Autodesk Inventor part; units mm, degrees
ref_plane "YZ Plane" through (0, 0, 0) normal (1, 0, 0) x (0, 1, 0)
ref_plane "XZ Plane" through (0, 0, 0) normal (0, 1, 0) x (-1, 0, 0)
ref_plane "XY Plane" through (0, 0, 0) normal (0, 0, 1) x (1, 0, 0)
ref_plane "Work Plane1" through (0, 0, 0) normal (0, 0, 1) x (1, 0, 0)
sketch "Sketch1" plane through (0, 0, 0) normal (0, 0, 1) x (1, 0, 0)
  circle A0 centre (103.8623, 15.35) radius 2.15 construction
  circle A1 centre (103.8623, -15.35) radius 2.15 construction
  line L0 (-103.8623, 20.35) -> (-103.8623, -20.35) construction
  line L1 (108.8623, -20.35) -> (-103.8623, -20.35) construction
  line L2 (108.8623, 20.35) -> (108.8623, -20.35) construction
  line L3 (-103.8623, 20.35) -> (108.8623, 20.35) construction
  circle A2 centre (59.3407, 0) radius 6.5 construction
  circle A3 centre (59.3407, 0) radius 7
  circle A4 centre (59.3407, 0) radius 24.5216 construction
  line L4 (34.8192, 0) -> (24.8192, 0) construction
  line L5 (24.8192, -20.35) -> (24.8192, 20.35)
  line L6 (24.8192, 20.35) -> (98.3623, 20.35)
  line L7 (98.8623, -20.35) -> (98.8623, 20.35) construction
  line L8 (98.3623, -20.35) -> (24.8192, -20.35)
  line L9 (95.8623, -23.35) -> (95.8623, 9.65)
  line L10 (95.3623, -20.35) -> (24.8192, -20.35)
  line L11 (98.8623, 9.65) -> (95.8623, 9.65)
  line L12 (98.8623, 20.35) -> (98.8623, -20.35)
  line L13 (98.3623, 10.15) -> (95.3623, 10.15)
  line L14 (95.3623, 10.15) -> (95.3623, -23.3504)
  line L15 (98.3623, 10.15) -> (98.3623, 20.35)
  point P0 (0, 0)
  point P1 (95.3623, -20.35)
  dimension "d0" = 0.5
  dimension "d1" = 10
  dimension "d15" = 0.5
  dimension "d16" = 0.5
  dimension "d17" = 0.5
extrude "Extrusion1" add sketch "Sketch1" along normal blind 5
sketch "Sketch2" plane through (24.8192, -20.35, 0) normal (-1, 0, 0) x (0, 0, 1)
  line L0 (80.8, 35.7) -> (75.8, 35.7) construction
  line L1 (80.8, 45.7) -> (80.8, 35.7) construction
  line L2 (51.1, 45.7) -> (80.8, 45.7) construction
  line L3 (51.1, -4.2229) -> (51.1, 45.7) construction
  line L4 (26.6, -4.2229) -> (51.1, -4.2229) construction
  line L5 (26.6, -16.2229) -> (26.6, -4.2229) construction
  line L6 (65.2, -16.2229) -> (26.6, -16.2229) construction
  line L7 (65.2, 40.7) -> (65.2, -16.2229) construction
  line L8 (75.8, 40.7) -> (65.2, 40.7) construction
  line L9 (75.8, 35.7) -> (75.8, 40.7) construction
  line L10 (38.6, -16.2229) -> (0, -16.2229)
  line L11 (0, -16.2229) -> (0, -4.2229)
  line L12 (5, -4.2229) -> (38.6, -4.2229)
  line L13 (38.6, -4.2229) -> (38.6, -16.2229)
  line L14 (38.6, -10.2229) -> (26.6, -10.2229) construction
  line L15 (0, 40.7) -> (0, 0) construction
  line L16 (0, 0) -> (5, 0) construction
  line L17 (5, 40.7) -> (5, 0) construction
  line L18 (0, 40.7) -> (5, 40.7) construction
  line L19 (5, 5) -> (0, 5)
  line L20 (0, -4.2229) -> (0, 5)
  line L21 (5, 5) -> (5, -4.2229)
  point P0 (0, 20.35)
  dimension "d11" = 5
extrude "Extrusion2" add sketch "Sketch2" against normal blind 5
equation "\"d15\" = d0"
equation "\"d16\" = d0"
equation "\"d17\" = d0"
equation "\"d9\" = d2"
equation "\"d11\" = d2"
equation "\"d12\" = d2"
properties part number "Button Bracket 2"
Here's how the part is built. I have some questions about the finished solid (model axes, mm). A direction names the side the tool comes from. Coordinates: 2 decimals unless noted, no trailing zeros. Order: outer loops, then holes, each group sorted by start corner. A loop starts at its lowest first (then second) coordinate and runs counter-clockwise, first axis right, second up. Notation, with made-up numbers: (41, 52.5) -> (51, 52.5) arc R9 ccw to (51, 62.5) -> close; hole circle Ø8 at (-10.75, 31). An arc over 180 degrees is marked (long way). Return JSON: item names as keys, results as strings.
1) If we section it at C-C on x = 57: List the corners of the cut face in (y, z) for me, plus the area to 3 significant figures.
Conclusion:
{"outline": "(-20.35, 0) -> (-6.6, 0) -> (-6.6, 5) -> (-20.35, 5) -> close; (6.6, 0) -> (20.35, 0) -> (20.35, 5) -> (6.6, 5) -> close", "area": "138 mm²"}
2) If I drill on probe 1 along X at (y, z) = (-29, 10); probe 2 along Y at (x, z) = (31, 3); probe 3 along Z at (x, y) = (74, -9.5), over which ranges is the centre line in solid material (lowest first)?
Conclusion:
{"probe 1": "x = 24.82 to 29.82", "probe 2": "y = -20.35 to 20.35", "probe 3": "z = 0 to 5"}
3) If we section it at D-D on z = 22: List the corners of the cut face in (x, y) for me, plus the area to 3 significant figures.
Conclusion:
{"outline": "(24.82, -36.57) -> (29.82, -36.57) -> (29.82, -24.57) -> (24.82, -24.57) -> close", "area": "60.0 mm²"}
4) I'm going to push flat-ended pins straight in: P1, Ø8, axis at y = -30.5, z = 24, coming from the +X side; P2, Ø1.5, axis at x = 63, y = -18.5, coming from the +Z side; P3, Ø1.5, axis at x = 97, z = 3.5, coming from the -Y side; P4, Ø5, axis at x = 33.5, z = 28, coming from the -Y side. Where does each tip first touch, or does it pass through?
Conclusion:
{"P1": "stops at x = 29.82", "P2": "stops at z = 5", "P3": "stops at y = 10.15", "P4": "passes through"}
5) If we section it at B-B on z = 4: List the corners of the cut face in (x, y) for me.
Conclusion:
{"outline": "(24.82, -36.57) -> (29.82, -36.57) -> (29.82, -20.35) -> (95.36, -20.35) -> (95.36, 10.15) -> (98.36, 10.15) -> (98.36, 20.35) -> (24.82, 20.35) -> close; hole circle Ø14 at (59.34, 0)"}
6) If we section it at A-A on y = 0: List the corners of the cut face in (x, z) for me, plus the area to 3 significant figures.
Conclusion:
{"outline": "(24.82, 0) -> (52.34, 0) -> (52.34, 5) -> (24.82, 5) -> close; (66.34, 0) -> (95.36, 0) -> (95.36, 5) -> (66.34, 5) -> close", "area": "283 mm²"}
7) Thinking about a two-plate mould opening in X: for faces 4 (the flat face through (24.819, -25, 15)), 5 (the flat face through (95.362, -5, 2)), 6 (the cylindrical face through (52.347, -0.308, 2.465)), 7 (the flat face through (27, -36.573, 20)), which applies, +X half, -X half, draft (parallel to the pull), parting line (faces both ways), or undercut?
Conclusion:
{"face 4": "-X half", "face 5": "+X half", "face 6": "undercut", "face 7": "draft"}
8) On a 3-axis mill with a long thin cutter (end or side, diameter ignored), from which of +Z, -Z, +X, -X, +Y, -Y can I reach the whole of each face in a straight line? I mean faces 1 (the flat face through (61, 20.35, 2)), 2 (the flat face through (27, -24.573, 22)), 3 (the flat face through (29.819, -30, 19)). Say none if no direction works.
Conclusion:
{"face 1": "+Z, -Z, +X, -X, +Y", "face 2": "+Z, +X, -X, +Y", "face 3": "+Z, -Z, +X, -Y"}
